The drawing under review shows one solid part. Ordinate dimensions are in mm from its lowest x, y, z. A direction names the side the tool comes from. Coordinates: 2 decimals unless noted, no trailing zeros. Order: outer loops, then holes, each group sorted by start corner. A loop starts at its lowest first (then second) coordinate and runs counter-clockwise, first axis right, second up. Notation, with made-up numbers: M 43.25,46 L 87.25,46 A19 cw 87.25,66 Z; hole C 47,25 d4. An arc over 180 degrees is marked long. Answer as a JSON object with one key per item and string values.
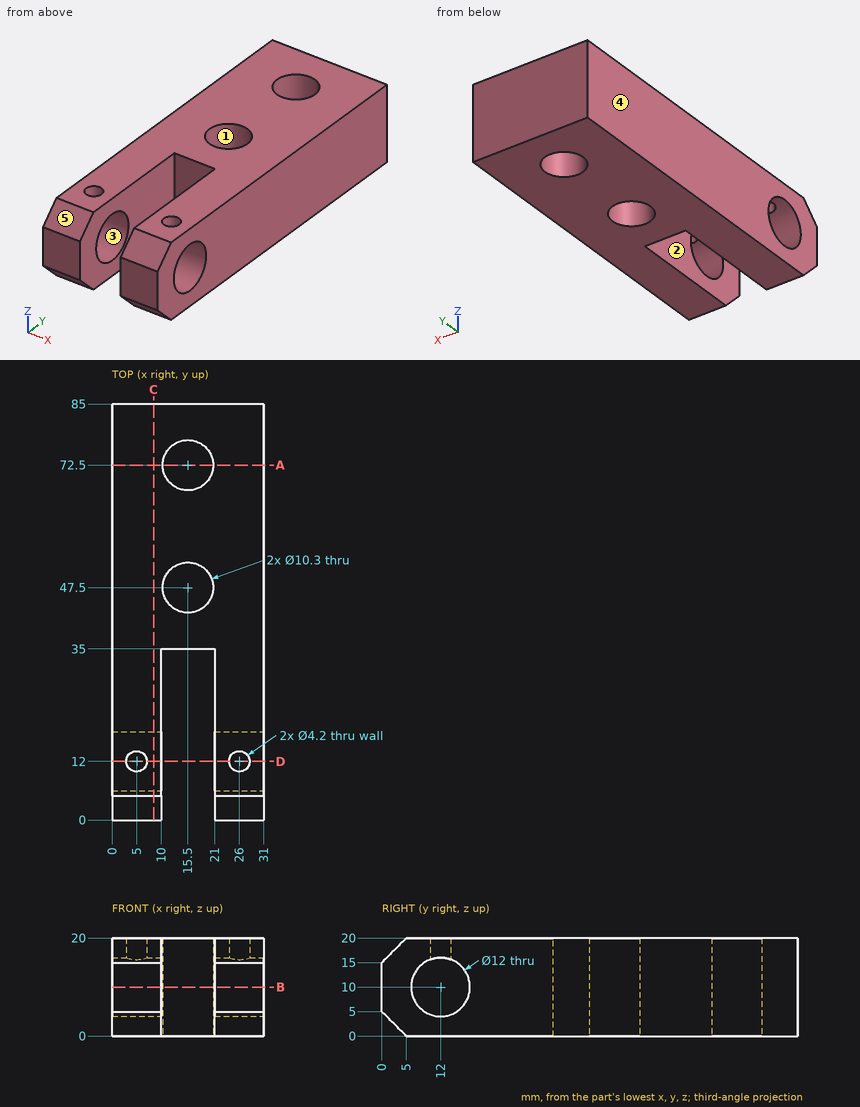
1) Add section D-D (y = 12). State the section outline as (x, z) points, and give its area (3 significant figures).
Taken from the geometry:
{"outline": "M 0,0 L 10,0 L 10,4 L 0,4 Z; M 0,16 L 2.9,16 L 2.9,20 L 0,20 Z; M 7.1,16 L 10,16 L 10,20 L 7.1,20 Z; M 21,0 L 31,0 L 31,4 L 21,4 Z; M 21,16 L 23.9,16 L 23.9,20 L 21,20 Z; M 28.1,16 L 31,16 L 31,20 L 28.1,20 Z", "area": "126 mm2"}
2) Insertion check: pin 1 Ø1 at (x, y) = (6, 13) entering from +Z. The pin has a flat end and moves straight along its axis. Give the tip position at first contact, or say it passes through.
Taken from the geometry:
{"pin 1": "stops at z = 4.19"}
3) Tool access review of the marked faces 1 and 2: name each direction out of +Z, -Z, +X, -X, +Y, -Y from which nothing blocks a thin tool from reaching the whole face with its end or side.
Taken from the geometry:
{"face 1": "+Z, -Z", "face 2": "+Z, -Z, -Y"}
4) Add section B-B (z = 10). State the section outline as (x, y) points, and give its area (3 significant figures).
Taken from the geometry:
{"outline": "M 0,0 L 10,0 L 10,6 L 0,6 Z; M 0,18 L 10,18 L 10,35 L 21,35 L 21,18 L 31,18 L 31,85 L 0,85 Z; M 21,0 L 31,0 L 31,6 L 21,6 Z; hole C 15.5,47.5 d10.3; hole C 15.5,72.5 d10.3", "area": "1,840 mm2"}
5) Mouldability with a two-part tool opening along Z and no side actions: class the marked faces 3, 4 and 5 as released by +Z, released by -Z, zero draft, split by the parting line, or undercut.
Taken from the geometry:
{"face 3": "undercut", "face 4": "zero draft", "face 5": "released by +Z"}
6) Add section C-C (x = 8.5). State the section outline as (y, z) points.
Taken from the geometry:
{"outline": "M 0,5 L 5,0 L 85,0 L 85,20 L 5,20 L 0,15 Z; hole C 12,10 d12"}
7) To check wall thickness, follow L1, parallel to Y at x = 15.5, z = 5.5; L2, parallel to X at y = 12, z = 16.75; L3, parallel to X at y = 25.5, z = 15.5. State the ranges of each line that lie inside material, in increasing order.
Taken from the geometry:
{"L1": "y = 35 to 42.35, 52.65 to 67.35, 77.65 to 85", "L2": "x = 0 to 2.9, 7.1 to 10, 21 to 23.9, 28.1 to 31", "L3": "x = 0 to 10, 21 to 31"}
8) Add section A-A (y = 72.5). State the section outline as (x, z) points.
Taken from the geometry:
{"outline": "M 0,0 L 10.35,0 L 10.35,20 L 0,20 Z; M 20.65,0 L 31,0 L 31,20 L 20.65,20 Z"}
